For this review, take the finished solid that the model builds, in its own axes (mm). A direction names the side the tool comes from. Give positions to 0.01 mm unless a question says otherwise; leave off trailing zeros. Order: outer loops, then holes, each group sorted by start corner. A loop starts at its lowest first (then second) coordinate and runs counter-clockwise, first axis right, second up.
from build123d import *

# Parameters (mm, degrees)
SKETCH1_W           = 280
SKETCH1_H           = 210
BOSS_EXTRUDE1_DEPTH = 15
SKETCH2_R           = 5
BOSS_EXTRUDE2_DEPTH = 50
SKETCH3_W           = 10
SKETCH3_H           = 30
BOSS_EXTRUDE3_DEPTH = 50
SKETCH4_R           = 13
CUT_EXTRUDE1_DEPTH  = 20
SKETCH5_W           = 360.4909063
SKETCH5_H           = 249.182613404
SKETCH5_W_2         = 248.173776912
SKETCH5_H_2         = 125.095724948
CUT_EXTRUDE5_DEPTH  = 15
CUT_EXTRUDE6_START  = -65
SKETCH7_R           = 5
CUT_EXTRUDE6_DEPTH  = 65
SKETCH9_W           = 29.33
SKETCH9_H           = 16.92
CUT_EXTRUDE9_DEPTH  = 148.681383345
SKETCH8_R           = 10.1
CUT_EXTRUDE11_DEPTH = 10
SKETCH11_W          = 17.231524428
SKETCH11_H          = 37.334969593
CUT_EXTRUDE13_DEPTH = 50
SKETCH15_W          = 10
SKETCH15_H          = 50
CUT_EXTRUDE14_DEPTH = 5
SKETCH13_W          = 26.98462743
SKETCH13_H          = 41.59552633
CUT_EXTRUDE17_DEPTH = 140.766916639
CUT_EXTRUDE18_DEPTH = 140.766916639


with BuildPart() as part:
    # Sketch1 → Boss-Extrude1 (new body)
    with BuildSketch(Plane(origin=(0, 0, 0), x_dir=(1, 0, 0), z_dir=(0, 1, 0))):
        Rectangle(SKETCH1_W, SKETCH1_H)
    extrude(amount=BOSS_EXTRUDE1_DEPTH)

    # Sketch2 → Boss-Extrude2 (add)
    with BuildSketch(Plane(origin=(0, 15, 0), x_dir=(1, 0, 0), z_dir=(0, 1, 0))):
        with Locations(Location((-100, 0, 0), (0, 0, 270))):
            Circle(SKETCH2_R)
        with Locations(Location((-100, 45, 0), (0, 0, 270))):
            Circle(SKETCH2_R)
        with Locations(Location((-100, -45, 0), (0, 0, 270))):
            Circle(SKETCH2_R)
    extrude(amount=BOSS_EXTRUDE2_DEPTH)

    # Sketch3 → Boss-Extrude3 (add)
    with BuildSketch(Plane(origin=(0, 15, 0), x_dir=(1, 0, 0), z_dir=(0, 1, 0))):
        Rectangle(SKETCH3_W, SKETCH3_H)
    extrude(amount=BOSS_EXTRUDE3_DEPTH)

    # Sketch4 → Cut-Extrude1 (cut)
    with BuildSketch(Plane(origin=(5, 0, 0), x_dir=(0, 0, -1), z_dir=(1, 0, 0))):
        with Locations((0, 41.236240869)):
            Circle(SKETCH4_R)
    extrude(amount=-CUT_EXTRUDE1_DEPTH, mode=Mode.SUBTRACT)

    # Sketch5 → Cut-Extrude5 (cut)
    with BuildSketch(Plane(origin=(0, 0, 0), x_dir=(1, 0, 0), z_dir=(0, 1, 0))):
        with Locations((1.345115322, -3.19464889)):
            Rectangle(SKETCH5_W, SKETCH5_H)
        Rectangle(SKETCH5_W_2, SKETCH5_H_2, mode=Mode.SUBTRACT)
    extrude(amount=CUT_EXTRUDE5_DEPTH, mode=Mode.SUBTRACT)

    # Sketch7 → Cut-Extrude6 (cut)
    with BuildSketch(Plane(origin=(0, 65, 0), x_dir=(1, 0, 0), z_dir=(0, 1, 0)).offset(CUT_EXTRUDE6_START)):
        with Locations(Location((-100, 45, 0), (0, 0, 270))):
            Circle(SKETCH7_R)
        with Locations(Location((-100, 0, 0), (0, 0, 270))):
            Circle(SKETCH7_R)
        with Locations(Location((-100, -45, 0), (0, 0, 270))):
            Circle(SKETCH7_R)
    extrude(amount=CUT_EXTRUDE6_DEPTH, mode=Mode.SUBTRACT)

    # Sketch9 → Cut-Extrude9 (cut, through all)
    with BuildSketch(Plane(origin=(0, 15, 0), x_dir=(1, 0, 0), z_dir=(0, 1, 0))):
        with Locations((-48.397782089, 47.087862474)):
            Rectangle(SKETCH9_W, SKETCH9_H)
    extrude(amount=-CUT_EXTRUDE9_DEPTH, mode=Mode.SUBTRACT)

    # Sketch8 → Cut-Extrude11 (cut)
    with BuildSketch(Plane.XZ):
        with Locations(Location((-100, 45, 0), (0, 0, 270))):
            Circle(SKETCH8_R)
        with Locations(Location((-100, 0, 0), (0, 0, 270))):
            Circle(SKETCH8_R)
        with Locations(Location((-100, -45, 0), (0, 0, 270))):
            Circle(SKETCH8_R)
    extrude(amount=-CUT_EXTRUDE11_DEPTH, mode=Mode.SUBTRACT)

    # Sketch11 → Cut-Extrude13 (cut)
    with BuildSketch(Plane(origin=(0, 65, 0), x_dir=(1, 0, 0), z_dir=(0, 1, 0))):
        with Locations((-3.002833284, 0.13632265)):
            Rectangle(SKETCH11_W, SKETCH11_H)
    extrude(amount=-CUT_EXTRUDE13_DEPTH, mode=Mode.SUBTRACT)

    # Sketch15 → Cut-Extrude14 (cut)
    with BuildSketch(Plane(origin=(0, 15, 0), x_dir=(1, 0, 0), z_dir=(0, 1, 0))):
        with Locations((-75, 0)):
            Rectangle(SKETCH15_W, SKETCH15_H)
    extrude(amount=-CUT_EXTRUDE14_DEPTH, mode=Mode.SUBTRACT)

    # Sketch13 → Cut-Extrude17 (cut, through all)
    with BuildSketch(Plane(origin=(0, 15, 0), x_dir=(1, 0, 0), z_dir=(0, 1, 0))):
        with Locations((46.507686285, 0.099999998)):
            Rectangle(SKETCH13_W, SKETCH13_H)
        with Locations((-56.507686285, 0.099999998)):
            Rectangle(SKETCH13_W, SKETCH13_H)
    extrude(amount=-CUT_EXTRUDE17_DEPTH, mode=Mode.SUBTRACT)

    # Sketch10 → Cut-Extrude18 (cut, through all)
    with BuildSketch(Plane(origin=(0, 15, 0), x_dir=(1, 0, 0), z_dir=(0, 1, 0))):
        Polygon((10.617962241, 13.45155831), (10.617962241, -16.40773575), (21.11227659, -7.629229077), (21.11227659, -32.023722987), (10.617962241, -26.54844169), (10.617962241, -56.40773575), (21.11227659, -47.629229077), (21.11227659, -62.347862477), (21.11227659, -67.048787633), (-140.704260322, -76.023181518), (-140.704260322, 77.849476584), (21.11227659, 83.143957129), (21.11227659, 62.347862473), (21.11227659, 47.976277013), (10.617962241, 53.45155831), (10.617962241, 23.59226425), (21.11227659, 32.370770923), (21.11227659, 7.976277013), align=None)
    extrude(amount=-CUT_EXTRUDE18_DEPTH, mode=Mode.SUBTRACT)


solid = part.part
1) To check wall thickness, follow line 1 (X direction, y = 13.75, z = -18); line 2 (Z direction, x = 38, y = 1.5); line 3 (X direction, y = 6.75, z = 15.5). State the ranges of each line that lie inside material, in increasing order.
Answer sheet:
line 1: x = 21.11 to 33.02, 60 to 124.09
line 2: z = -62.55 to -20.9, 20.7 to 62.55
line 3: x = 10.62 to 11.7, 21.11 to 33.02, 60 to 124.09
2) We need section D-D on z = -11.5. Give the boundary of the cut face in (x, y).
Answer sheet:
outline: (10.62, 0) - (14.36, 0) - (14.36, 15) - (10.62, 15) - close; (21.11, 0) - (33.02, 0) - (33.02, 15) - (21.11, 15) - close; (60, 0) - (124.09, 0) - (124.09, 15) - (60, 15) - close
3) Tool access review of faces 4 (the face through (21.112, 8, 55)), 5 (the face through (15.939, 7.605, -10.676)), 6 (the face through (15.939, 7.605, -50.676)): name each direction out of +Z, -Z, +X, -X, +Y, -Y from which nothing blocks a thin tool from reaching the whole face with its end or side.
Answer sheet:
face 4: +Z, +Y, -Y
face 5: +Y, -Y
face 6: -Z, +Y, -Y
4) Draft analysis for pull direction Z (two halves, no side actions). For faces 1 (the face through (15.79, 7.6, 52.08)), 2 (the face through (46, 8, 20.698)), 3 (the face through (67, 0, -1)), state which applies: +Z half, -Z half, draft (parallel to the pull), parting line (faces both ways), or undercut.
Answer sheet:
face 1: +Z half
face 2: undercut
face 3: draft
5) We need section A-A on y = 7.25. Give the boundary of the cut face in (x, z).
Answer sheet:
outline: (10.62, -53.45) - (21.11, -47.98) - (21.11, -62.55) - (124.09, -62.55) - (124.09, 62.55) - (21.11, 62.55) - (21.11, 47.63) - (10.62, 56.41) - (10.62, 26.55) - (21.11, 32.02) - (21.11, 7.63) - (10.62, 16.41) - (10.62, -13.45) - (21.11, -7.98) - (21.11, -32.37) - (10.62, -23.59) - close; hole (33.02, -20.9) - (60, -20.9) - (60, 20.7) - (33.02, 20.7) - close
6) We need section C-C on z = -26. Give the boundary of the cut face in (x, y), then the cut area to 3 significant figures.
Answer sheet:
outline: (10.62, 0) - (13.5, 0) - (13.5, 15) - (10.62, 15) - close; (21.11, 0) - (124.09, 0) - (124.09, 15) - (21.11, 15) - close
area: 1,590 mm2
7) Clearance check with a flat-ended pin moving along its axis: pin 1 (7.5 mm diameter, centred on y = 10.5, z = -56, fed in from -X). State where the tip first meets the part, or that it passes through.
Answer sheet:
pin 1: stops at x = 10.62
8) We need section B-B on x = 45. Give the boundary of the cut face in (y, z), then the cut area to 3 significant figures.
Answer sheet:
outline: (0, -62.55) - (15, -62.55) - (15, -20.9) - (0, -20.9) - close; (0, 20.7) - (15, 20.7) - (15, 62.55) - (0, 62.55) - close
area: 1,250 mm2
